For this review, take the finished solid that the model builds, in its own axes (mm). Give positions to 0.01 mm unless a question says otherwise; leave off trailing zeros. Write each loop counter-clockwise with the first axis right and the second up, starting at its lowest first coordinate (ties: lowest second). Pieces come first, ordered by that corner, then holes. Notation, with made-up numbers: (-6.75, 78.25) -> (34.25, 78.25) arc R28 ccw to (34.25, 101.25) -> close; hole circle Ø7 at (40.25, -26.75). An arc over 180 degrees is marked (long way). Return JSON: item names as keys, results as strings.
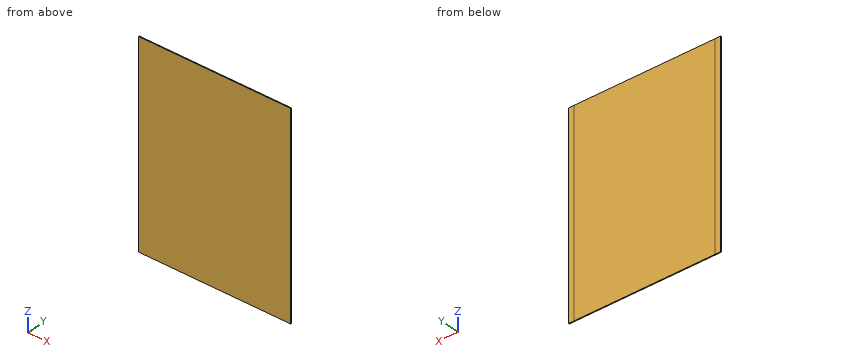
Autodesk Inventor part; units mm, degrees
ref_plane "YZ Plane" through (0, 0, 0) normal (1, 0, 0) x (0, 1, 0)
ref_plane "XZ Plane" through (0, 0, 0) normal (0, 1, 0) x (-1, 0, 0)
ref_plane "XY Plane" through (0, 0, 0) normal (0, 0, 1) x (1, 0, 0)
sketch "Sketch1" plane through (0, 0, 0) normal (0, 1, 0) x (-1, 0, 0)
  line L0 (275, 0) -> (-275, 0)
  line L1 (-275, 0) -> (-275, -720)
  line L2 (-275, -720) -> (275, -720)
  line L3 (275, -720) -> (275, 0)
  line L4 (255, 0) -> (255, -720)
  line L5 (-255, -720) -> (-255, 0)
  point P0 (0, 0)
  point P1 (0, 0)
  dimension "d0" = 550
  dimension "d1" = 720
  dimension "d4" = 20
  dimension "d5" = 20
extrude "Extrusion1" add sketch "Sketch1" along normal blind 3
extrude "Extrusion2" add sketch "Sketch1" along normal blind 3.1 contours L3 L2 L4 L0 | L5 L2 L1 L0
equation "\"d0\" = track_width"
equation "\"d4\" = curb_width"
equation "\"d5\" = curb_width"
equation "\"d2\" = track_height"
equation "\"d6\" = track_height + curb_height"
properties part number "straight"
1. Add section B-B, the plane x = 108. State the section outline as (y, z) points.
Results found:
{"outline": "(0, -720) -> (3, -720) -> (3, 0) -> (0, 0) -> close"}
2. To check wall thickness, follow probe 1 along Y at (x, z) = (121, -627). State the ranges of the line that lie inside material, in increasing order.
Results found:
{"probe 1": "y = 0 to 3"}
3. For pin 1 (1.5 mm diameter, centred on x = -177.5, y = 2, fed in from +Z); pin 2 (4 mm diameter, centred on x = 15, z = -424, fed in from +Y), all flat-tipped, find the tip position at first contact; note any pin that passes through.
Results found:
{"pin 1": "stops at z = 0", "pin 2": "stops at y = 3"}
4. Add section A-A, the plane z = -257. State the section outline as (x, y) points.
Results found:
{"outline": "(-275, 0) -> (275, 0) -> (275, 3.1) -> (255, 3.1) -> (255, 3) -> (-255, 3) -> (-255, 3.1) -> (-275, 3.1) -> close"}
